Could you check a few things on this model? Use its own coordinates, in mm. A direction names the side the tool comes from. Coordinates: 2 decimals unless noted, no trailing zeros. Loops run counter-clockwise (first coordinate to the right, second up) from the corner with the lowest first, then second, coordinate; pieces in that order, holes last.
1) If I drill on line 1 along X through (y, z) = (-0.75, 0.25) (3 decimals); line 2 along Z through (x, y) = (8.5, -0.05); line 3 along X through (y, z) = (-0.5, -2) (3 decimals), over which ranges is the centre line in solid material (lowest first)?
2) For faces 1 (the face through (2.125, -2.44, -1.4)), 2 (the face through (2.625, -2, 0)), 3 (the face through (2.125, -2.44, 1.41)), 4 (the face through (2.125, 2.44, -1.4)), 5 (the face through (1.048, -1.311, 2.314)), which set-ups out of +Z, -Z, +X, -X, +Y, -Y let a thin tool reach every point of the face, with its end or its side?
3) Thinking about a two-plate mould opening in Z: for faces 6 (the face through (1.048, 1.311, -2.314)), 7 (the face through (12.35, 0.07, 1.5)), 8 (the face through (0.7, 0, 0)), which applies, released by +Z, released by -Z, zero draft, split by the parting line, or undercut?
4) Will these pins go through, and if not, where does the flat tip stop? P1, Ø2, axis at y = 0, z = -1.5, coming from the -X side; P2, Ø0.6, axis at y = 0, z = -3, coming from the +X side (3 decimals); P3, Ø0.8, axis at x = 0.5, y = 1, coming from the -Z side; P4, Ø1.1, axis at y = 2, z = -1.5, coming from the +X side (3 decimals).
5) Imagine slicing it at A-A on x = 8. Please give me the cut outline in (y, z).
```python
from build123d import *

# Parameters (mm, degrees)
BASEHEAD_DEPTH  = 2.125
SKETCH3_R       = 1.5
BASEBODY_DEPTH  = 20
CHAMFER1_SIZE   = 0.2705
SLOT_DEPTH      = 23.986960615
SLOT_DEPTH_BACK = 23.986960615
SKETCH5_W       = 0.7
SKETCH5_H       = 0.8


with BuildPart() as part:
    # Sketch-BaseHead → BaseHead (new body)
    with BuildSketch(Plane(origin=(0, 0, 0), x_dir=(0, 0, -1), z_dir=(1, 0, 0))):
        Polygon((1.535751716, -2.66), (3.071503432, 0), (1.535751716, 2.66), (-1.535751716, 2.66), (-3.071503432, 0), (-1.535751716, -2.66), align=None)
    extrude(amount=BASEHEAD_DEPTH)

    # Sketch1 → Revolve1 (revolve)
    with BuildSketch(Plane.XY, mode=Mode.PRIVATE) as revolve1_sk:
        Polygon((2.125, 0), (2.625, 0), (2.625, -2.285), (2.125, -2.66), align=None)
    revolve(revolve1_sk.sketch.rotate(Axis((-4.001564945, 0, 0), (1, 0, 0)), 270), axis=Axis((-4.001564945, 0, 0), (1, 0, 0)))

    # Sketch3 → BaseBody (add)
    with BuildSketch(Plane(origin=(2.625, 0, 0), x_dir=(0, 0, -1), z_dir=(1, 0, 0))):
        Circle(SKETCH3_R)
    extrude(amount=BASEBODY_DEPTH)

    # Chamfer1
    chamfer1_edges = [part.edges().sort_by_distance(p)[0] for p in [
        (22.625, 0, 1.5),
    ]]
    chamfer(chamfer1_edges, length=CHAMFER1_SIZE)

    # Sketch4 → HeadChamfer (revolve, cut)
    with BuildSketch(Plane(origin=(-0.264637255, 0, 5.916896391), x_dir=(0, 0, -1), z_dir=(0, 1, 0)), mode=Mode.PRIVATE) as headchamfer_sk:
        Polygon((8.988399823, -0.264637255), (8.576896391, -0.264637255), (8.988399823, -0.414412256), align=None)
    revolve(headchamfer_sk.sketch.rotate(Axis((-4.001564945, 0, 0), (1, 0, 0)), 180), axis=Axis((-4.001564945, 0, 0), (1, 0, 0)), mode=Mode.SUBTRACT)

    # Sketch5 → Slot (cut, two sides: drawn at the far end of the back side and taken through both)
    with BuildSketch(Plane(origin=(0, 0, 0), x_dir=(1, 0, 0), z_dir=(0, 1, 0)).offset(-SLOT_DEPTH_BACK)):
        with Locations((0.35, 0)):
            Rectangle(SKETCH5_W, SKETCH5_H)
    extrude(amount=SLOT_DEPTH + SLOT_DEPTH_BACK, mode=Mode.SUBTRACT)


solid = part.part
```
Filled in:
1. line 1: x = 0.7 to 22.625
1. line 2: z = -1.5 to 1.5
1. line 3: x = 0 to 2.625
2. face 1: -Z, +X, -Y
2. face 2: +X
2. face 3: +Z, +X, -Y
2. face 4: -Z, +X, +Y
2. face 5: +Z, +X, -X, -Y
3. face 6: released by -Z
3. face 7: split by the parting line
3. face 8: undercut
4. P1: stops at x = 0
4. P2: stops at x = 2.125
4. P3: stops at z = -2.73
4. P4: stops at x = 2.625
5. outline: circle Ø3 at (0, 0)
